Input: part model. Units: mm. Frame: model coordinates. A direction names the side the tool comes from. Give positions to 0.01 mm unless a question says otherwise; leave off trailing zeros. Order: outer loops, then holes, each group sorted by start corner. A loop starts at its lowest first (then second) coordinate and runs counter-clockwise, first axis right, second up. Notation, with made-up numbers: (11.5, 56) - (66.5, 56) arc R32 ccw to (66.5, 87) - close; hole circle Ø1 at (-6, -1.5). An arc over 180 degrees is marked (long way). Answer in a Markdown table with one row per item. Add a question column.
1. Mould query, pull axis Y, two halves, no side actions, for faces 1 (the face through (-8.31, 4.71, 5.92)), 2 (the face through (-14.985, 0.66, 17.255)), 3 (the face through (3, 15, 35)). Classes: released by +Y, released by -Y, zero draft, split by the parting line, or undercut.
2. Ray query, line 1 (Y direction, x = 0, z = 40); line 2 (Y direction, x = 0, z = 27.75). Return the intervals inside material, ascending. Write a range as [from, to].
3. Section query B-B on z = 7. Return loops of the section in (x, y).
4. Section query C-C on y = 5. Return loops of the section in (x, z), and give its area (3 significant figures).
5. Section query D-D on x = -16. Return loops of the section in (y, z).
6. Contact query for flat-ended pins moving along their axis: pin 1 (6 mm diameter, centred on y = 14, z = 38, fed in from +X); pin 2 (3.5 mm diameter, centred on x = -0.5, z = 5.5, fed in from -Y); pin 3 (8 mm diameter, centred on x = -15, y = -10, fed in from +Z); pin 4 (4 mm diameter, centred on x = 0, y = 2, fed in from -Z). Output: stop coordinate, or through.
7. Access query for faces 4 (the face through (-6, 0, 40)), 5 (the face through (0, -9.55, 6)). Directions: +Z, -Z, +X, -X, +Y, -Y. A direction counts if a zero-diameter tool reaches every point of the face in a straight line with its end or side. Return the directions, or none.
8. Section query A-A on x = 0. Return loops of the section in (y, z).
```python
from build123d import *

# Parameters (mm, degrees)
SKETCH1_R                    = 15
BOSS_EXTRUDE1_DEPTH          = 35
CUT_EXTRUDE1_DEPTH           = 12
F_12_5_12_5_DIAMETER_HOLE1_D = 12.5
SKETCH10_R                   = 20
SKETCH10_R_2                 = 6
BOSS_EXTRUDE2_DEPTH          = 10


with BuildPart() as part:
    # Sketch1 → Boss-Extrude1 (new body)
    with BuildSketch(Plane.XY):
        Circle(SKETCH1_R)
    extrude(amount=BOSS_EXTRUDE1_DEPTH)

    # Sketch5 → Cut-Extrude1 (cut)
    with BuildSketch(Plane(origin=(0, 0, 0), x_dir=(-1, 0, 0), z_dir=(0, 0, -1))):
        Polygon((11.027390142, 0), (5.513695071, 9.55), (-5.513695071, 9.55), (-11.027390142, 0), (-5.513695071, -9.55), (5.513695071, -9.55), align=None)
    extrude(amount=-CUT_EXTRUDE1_DEPTH, mode=Mode.SUBTRACT)

    # Ø12.5 (12.5) Diameter Hole1 (through all)
    with Locations(Plane(origin=(0, 0, 12), x_dir=(-1, 0, 0), z_dir=(0, 0, -1))):
        with Locations((0, 0)):
            Hole(F_12_5_12_5_DIAMETER_HOLE1_D / 2)

    # Sketch10 → Boss-Extrude2 (add)
    with BuildSketch(Plane.XY.offset(35)):
        Circle(SKETCH10_R)
        Circle(SKETCH10_R_2, mode=Mode.SUBTRACT)
    extrude(amount=BOSS_EXTRUDE2_DEPTH)

    # Sketch11 → Cut-Revolve6 (revolve, cut)
    with BuildSketch(Plane(origin=(0, 0, 0), x_dir=(1, 0, 0), z_dir=(0, 1, 0))):
        with BuildLine():
            Line((-20, -42.979589711), (-20, -45))
            Line((-20, -45), (-6, -45))
            Line((-6, -45), (-6, -44.819837708))
            ThreePointArc((-6, -44.819837708), (-13.032521942, -44.147129922), (-20, -42.979589711))
        make_face()
    revolve(axis=Axis((0, 0, 0), (0, 0, 1)), mode=Mode.SUBTRACT)


solid = part.part
```
Answer:
| question | item | result |
|---|---|---|
| 1 | face 1 | undercut |
| 1 | face 2 | split by the parting line |
| 1 | face 3 | zero draft |
| 2 | line 1 | y = [-20, -6], [6, 20] |
| 2 | line 2 | y = [-15, -6.25], [6.25, 15] |
| 3 | outline | circle Ø30 at (0, 0); hole (-11.03, 0) - (-5.51, -9.55) - (5.51, -9.55) - (11.03, 0) - (5.51, 9.55) - (-5.51, 9.55) - close |
| 4 | outline | (-19.36, 35) - (-14.14, 35) - (-14.14, 0) - (-8.14, 0) - (-8.14, 12) - (-3.75, 12) - (-3.75, 35) - (-3.32, 35) - (-3.32, 44.82) arc R99.87 ccw to (-19.36, 42.98) - close; (3.32, 35) - (3.75, 35) - (3.75, 12) - (8.14, 12) - (8.14, 0) - (14.14, 0) - (14.14, 35) - (19.36, 35) - (19.36, 42.98) arc R99.87 ccw to (3.32, 44.82) - close |
| 4 | area | 915 mm² |
| 5 | outline | (-12, 35) - (12, 35) - (12, 42.98) arc R98.71 ccw to (-12, 42.98) - close |
| 6 | pin 1 | stops at x = 16.7 |
| 6 | pin 2 | stops at y = -15 |
| 6 | pin 3 | stops at z = 44.01 |
| 6 | pin 4 | passes through |
| 7 | face 4 | +Z, -Z |
| 7 | face 5 | -Z |
| 8 | outline | (-20, 35) - (-15, 35) - (-15, 0) - (-9.55, 0) - (-9.55, 12) - (-6.25, 12) - (-6.25, 35) - (-6, 35) - (-6, 44.82) arc R100 ccw to (-20, 42.98) - close; (6, 35) - (6.25, 35) - (6.25, 12) - (9.55, 12) - (9.55, 0) - (15, 0) - (15, 35) - (20, 35) - (20, 42.98) arc R100 ccw to (6, 44.82) - close |
